```python
from build123d import *


with BuildPart() as part:
    # Sketch1 → Revolve1 (revolve)
    with BuildSketch(Plane(origin=(0, 0, 0), x_dir=(0, 0, -1), z_dir=(1, 0, 0))):
        with BuildLine():
            Line((-15, 0), (-15, -10.35))
            Line((-15, -10.35), (-19, -10.35))
            Line((-19, -10.35), (-19, -4))
            Line((-19, -4), (-24, -4))
            Line((-24, -4), (-24, 2.493733733))
            Line((-24, 2.493733733), (-17.9, 0.8018))
            add(Edge.make_bspline(
                [(-15, 0), (-15.033336467, 0.009188668), (-15.100017964, 0.027568365), (-15.199979517, 0.055340747), (-15.300021158, 0.082856812), (-15.399978661, 0.110643842), (-15.500021387, 0.138155983), (-15.5999786, 0.165944064), (-15.700021404, 0.193455923), (-15.799978595, 0.22124408), (-15.900021405, 0.24875592), (-15.999978596, 0.276544077), (-16.1000214, 0.304055936), (-16.199978613, 0.331844017), (-16.300021339, 0.359356158), (-16.399978842, 0.387143188), (-16.500020483, 0.414659253), (-16.599982036, 0.442431635), (-16.7, 0.47), (-16.800017964, 0.497568365), (-16.899979517, 0.525340747), (-17.000021158, 0.552856812), (-17.099978661, 0.580643841), (-17.200021386, 0.608155987), (-17.299978604, 0.635944047), (-17.400021386, 0.663455987), (-17.499978661, 0.691243841), (-17.600021158, 0.718756812), (-17.699979517, 0.746540746), (-17.800017964, 0.774068364), (-17.866669801, 0.79255533), (-17.9, 0.8018)],
                knots=[0, 0, 0, 0, 0.034478483, 0.068965823, 0.103444305, 0.137931645, 0.172410128, 0.206897468, 0.241375951, 0.275863291, 0.310341773, 0.344829113, 0.379307596, 0.413794936, 0.448273419, 0.482760759, 0.517239241, 0.551726581, 0.586205064, 0.620683547, 0.655170887, 0.689649369, 0.724136709, 0.758615192, 0.793102532, 0.827581015, 0.862068355, 0.896546837, 0.931034177, 0.96551266, 1, 1, 1, 1], degree=3))
        make_face()
    revolve(axis=Axis((0, 0, 0), (0, -1, 0)))


solid = part.part
```
The listing builds one solid part. Answer for the finished solid, in the listing's coordinates (mm). Give positions to 0.01 mm unless a question says otherwise; leave off trailing zeros. Order: outer loops, then holes, each group sorted by start corner. A loop starts at its lowest first (then second) coordinate and runs counter-clockwise, first axis right, second up. Notation, with made-up numbers: M 57.5,23.25 L 106.5,23.25 A19 cw 106.5,33.25 Z; hole C 15.5,24.25 d3. An arc over 180 degrees is marked long. Put each result on its own line as item: value. Start each with the question number.
Item 1: For a pull along X with two mould halves and no side action, classify faces 1 (the face through (-0.66, -5.247, -14.985)), 2 (the face through (16.856, -7.131, 8.767)), 3 (the face through (-7, -4, -18)), 4 (the face through (16.143, 0.884, 8.396)) as +X half, -X half, draft (parallel to the pull), parting line (faces both ways), or undercut.
Item 2: The part is cut by section B-B, the plane y = -2.5. Determine the outline of the cut face in (x, z).
Item 3: Flat-ended cylindrical pins translate along their axes: P1, Ø3, axis at x = -5, y = -4.5, coming from the +Z side; P2, Ø1, axis at x = -12.5, z = -11.5, coming from the +Y side; P3, Ø2, axis at x = -18, z = -14, coming from the -Y side. Find the tip coordinate at first contact, or state that the pin passes through.
Item 4: Find the intervals of material crossed by line 1 along X through (y, z) = (-5.5, 0); line 2 along X through (y, z) = (-3.75, 0), in increasing order.
Item 5: The part is cut by section A-A, the plane y = -7.5. Determine the outline of the cut face in (x, z).
Answer key:
1. face 1: undercut
1. face 2: parting line
1. face 3: draft
1. face 4: undercut
2. outline: C 0,0 d48; hole C 0,0 d30
3. P1: stops at z = 23.73
3. P2: stops at y = 0.69
3. P3: stops at y = -4
4. line 1: x = -19 to -15, 15 to 19
4. line 2: x = -24 to -15, 15 to 24
5. outline: C 0,0 d38; hole C 0,0 d30
